```python
from build123d import *

# Parameters (mm, degrees)
SALIENTE_EXTRUIR1_DEPTH    = 40
CROQUIS3_R                 = 1.5
CORTAR_EXTRUIR2_DEPTH      = 40
CROQUIS2_W                 = 15
CROQUIS2_H                 = 20
CORTAR_EXTRUIR1_DEPTH      = 20
CORTAR_EXTRUIR3_DEPTH      = 44.084219849
CORTAR_EXTRUIR3_DEPTH_BACK = 44.084219849
CROQUIS4_R                 = 1.5
CORTAR_EXTRUIR4_DEPTH      = 44.08422
CORTAR_EXTRUIR4_DEPTH_BACK = 44.08422
CORTAR_EXTRUIR5_DEPTH      = 44.084220001
CORTAR_EXTRUIR5_DEPTH_BACK = 44.084220001
CUT_EXTRUDE1_DEPTH         = 4
SKETCH2_R                  = 3
BOSS_EXTRUDE1_DEPTH        = 2
SKETCH3_R                  = 4
BOSS_EXTRUDE2_DEPTH        = 2
FILLET1_R                  = 1
FILLET2_R                  = 1
FILLET3_R                  = 1


with BuildPart() as part:
    # Croquis1 → Saliente-Extruir1 (new body)
    with BuildSketch(Plane.XY):
        with BuildLine():
            Line((-10, 10), (10, 10))
            ThreePointArc((10, 10), (12.5, 0), (10, -10))
            Line((10, -10), (-10, -10))
            ThreePointArc((-10, -10), (-12.5, 0), (-10, 10))
        make_face()
    extrude(amount=SALIENTE_EXTRUIR1_DEPTH)

    # Croquis3 → Cortar-Extruir2 (cut)
    with BuildSketch(Plane(origin=(0, 0, 0), x_dir=(-1, 0, 0), z_dir=(0, 0, -1))):
        with Locations((0, -7)):
            Circle(CROQUIS3_R)
    extrude(amount=-CORTAR_EXTRUIR2_DEPTH, mode=Mode.SUBTRACT)

    # Croquis2 → Cortar-Extruir1 (cut)
    with BuildSketch(Plane(origin=(0, 0, 0), x_dir=(-1, 0, 0), z_dir=(0, 0, -1))):
        Rectangle(CROQUIS2_W, CROQUIS2_H)
    extrude(amount=-CORTAR_EXTRUIR1_DEPTH, mode=Mode.SUBTRACT)

    # Croquis4 → Cortar-Extruir3 (cut, two sides: drawn at the far end of the back side and taken through both)
    with BuildSketch(Plane(origin=(0, 0, 0), x_dir=(0, 0, -1), z_dir=(1, 0, 0)).offset(-CORTAR_EXTRUIR3_DEPTH_BACK)):
        with Locations((-10, 0)):
            Circle(CROQUIS4_R)
        with BuildLine():
            Line((-10, -10), (3, -10))
            Line((3, -10), (3, 10))
            Line((3, 10), (-10, 10))
            ThreePointArc((-10, 10), (0, 0), (-10, -10))
        make_face()
    extrude(amount=CORTAR_EXTRUIR3_DEPTH + CORTAR_EXTRUIR3_DEPTH_BACK, mode=Mode.SUBTRACT)

    # Croquis5 → Cortar-Extruir4 (cut, two sides: drawn at the far end of the back side and taken through both)
    with BuildSketch(Plane(origin=(0, 0, 0), x_dir=(1, 0, 0), z_dir=(0, 1, 0)).offset(-CORTAR_EXTRUIR4_DEPTH_BACK)):
        with BuildLine():
            Line((-12.5, -20), (-12.5, -42))
            Line((-12.5, -42), (12.5, -42))
            Line((12.5, -42), (12.5, -20))
            add(Edge.make_bspline(
                [(-12.5, -20), (-12.5, -40), (0, -40), (12.5, -40), (12.5, -20)],
                knots=[4.71238898, 4.71238898, 4.71238898, 6.283185307, 6.283185307, 7.853981634, 7.853981634, 7.853981634], degree=2, weights=[1, 0.707106781, 1, 0.707106781, 1]))
        make_face()
    extrude(amount=CORTAR_EXTRUIR4_DEPTH + CORTAR_EXTRUIR4_DEPTH_BACK, mode=Mode.SUBTRACT)

    # Croquis6 → Cortar-Extruir5 (cut, two sides: drawn at the far end of the back side and taken through both)
    with BuildSketch(Plane(origin=(0, 0, 0), x_dir=(0, 0, -1), z_dir=(1, 0, 0)).offset(-CORTAR_EXTRUIR5_DEPTH_BACK)):
        with BuildLine():
            Line((-20, 10), (-42, 10))
            Line((-42, 10), (-42, -10))
            Line((-42, -10), (-20, -10))
            add(Edge.make_bspline(
                [(-20, 10), (-40, 10), (-40, 0), (-40, -10), (-20, -10)],
                knots=[4.71238898, 4.71238898, 4.71238898, 6.283185307, 6.283185307, 7.853981634, 7.853981634, 7.853981634], degree=2, weights=[1, 0.707106781, 1, 0.707106781, 1]))
        make_face()
    extrude(amount=CORTAR_EXTRUIR5_DEPTH + CORTAR_EXTRUIR5_DEPTH_BACK, mode=Mode.SUBTRACT)

    # Sketch1 → Cut-Extrude1 (cut)
    with BuildSketch(Plane(origin=(0, 10, 0), x_dir=(1, 0, 0), z_dir=(0, 1, 0))):
        with BuildLine():
            Line((-6, -26), (-6, -20))
            Line((-6, -20), (6, -20))
            Line((6, -20), (6, -26))
            ThreePointArc((6, -26), (0, -32), (-6, -26))
        make_face()
    extrude(amount=-CUT_EXTRUDE1_DEPTH, mode=Mode.SUBTRACT)

    # Sketch2 → Boss-Extrude1 (add)
    with BuildSketch(Plane(origin=(0, 6, 0), x_dir=(1, 0, 0), z_dir=(0, 1, 0))):
        with Locations(Location((0, -26, 0), (0, 0, 270))):
            Circle(SKETCH2_R)
    extrude(amount=BOSS_EXTRUDE1_DEPTH)

    # Sketch3 → Boss-Extrude2 (add)
    with BuildSketch(Plane(origin=(0, 8, 0), x_dir=(1, 0, 0), z_dir=(0, 1, 0))):
        with Locations(Location((0, -26, 0), (0, 0, 270))):
            Circle(SKETCH3_R)
    extrude(amount=BOSS_EXTRUDE2_DEPTH)

    # Fillet1
    fillet1_edges = [part.edges().sort_by_distance(p)[0] for p in [
        (0, 6, 23),
        (0, 8, 23),
    ]]
    fillet(fillet1_edges, radius=FILLET1_R - 0.0001)  # a hair under: the kernel refuses the full size

    # Fillet2
    fillet2_edges = [part.edges().sort_by_distance(p)[0] for p in [
        (0, 6, 20),
    ]]
    fillet(fillet2_edges, radius=FILLET2_R)

    # Fillet3
    fillet3_edges = [part.edges().sort_by_distance(p)[0] for p in [
        (1.5, -7, 20),
    ]]
    fillet(fillet3_edges, radius=FILLET3_R)


solid = part.part
```
Verification items for the finished model (mm, model axes). A direction names the side the tool comes from. Give positions to 0.01 mm unless a question says otherwise; leave off trailing zeros. Write each loop counter-clockwise with the first axis right and the second up, starting at its lowest first coordinate (ties: lowest second). Pieces come first, ordered by that corner, then holes. Notation, with made-up numbers: M 78.25,41.25 L 126.25,41.25 A11 cw 126.25,47.25 Z; hole C -4,-9.5 d11. An arc over 180 degrees is marked long. One line per question, with ' | ' between items.
1) Thickness scan on line 1 along Y through (x, z) = (-9.95, 10); line 2 along X through (y, z) = (9, 28.5); line 3 along X through (y, z) = (-6, 16). Record the ranges inside material, lowest first. Write a range as [from, to].
Result:
line 1: y = [-10, -1.5], [1.5, 10] | line 2: x = [-10.5, -5.45], [-3.12, 3.12], [5.45, 10.5] | line 3: x = [-11.64, -7.5], [7.5, 11.64]
2) Section check A-A on z = 11. Enter the section's corners in (x, y).
Result:
outline: M -12.47,-1.12 A21.25 ccw -10,-10 L -7.5,-10 L -7.5,-1.12 Z; M -12.47,1.12 L -7.5,1.12 L -7.5,10 L -10,10 A21.25 ccw Z; M 7.5,-10 L 10,-10 A21.25 ccw 12.47,-1.12 L 7.5,-1.12 Z; M 7.5,1.12 L 12.47,1.12 A21.25 ccw 10,10 L 7.5,10 Z
3) Section check B-B on z = 29.5. State how many separate pieces and enclosed holes the cut face has, plus the area to 3 significant figures.
Result:
separate pieces: 2 | enclosed holes: 1 | area: 360 mm2
4) Set-up check for faces 5 (the flat face through (-6, 8, 23)), 6 (the cylindrical face through (-2.4, 9, 22.8)), 7 (the flat face through (0, 0, 20)): record each of +Z, -Z, +X, -X, +Y, -Y from which the full face is reachable in a straight line by a thin tool's end or side.
Result:
face 5: -Z, +Y | face 6: +Y | face 7: -Z, +Y, -Y
5) Gauge pin test, flat ends, axial feed: pin 1 Ø10 at (y, z) = (-5.5, 12.5) entering from -X; pin 2 Ø2.5 at (y, z) = (8.5, 22.5) entering from -X (3 decimals); pin 3 Ø7.5 at (x, y) = (-2, 0.5) entering from -Z; pin 4 Ø5 at (x, y) = (1.5, -2) entering from +Z. Record the tip position at first contact, or that the pin passes through.
Result:
pin 1: stops at x = -12.49 | pin 2: stops at x = -11.225 | pin 3: stops at z = 20 | pin 4: stops at z = 40
6) Mould release check, pull along Y, two halves, no side actions. Record for faces 1 (the flat face through (-9, -10, 15)), 2 (the flat face through (-7.5, 0, 12)), 3 (the cylindrical face through (-10.04, 0.07, 11.5)), 4 (the cylindrical face through (9, 0, 0)): released by +Y, released by -Y, zero draft, split by the parting line, or undercut.
Result:
face 1: released by -Y | face 2: zero draft | face 3: undercut | face 4: split by the parting line
